Drawing for the job (mm, zero at the part's lowest x, y, z). Give positions to 0.01 mm unless a question says otherwise; leave off trailing zeros. Order: outer loops, then holes, each group sorted by start corner. A loop starts at its lowest first (then second) coordinate and runs counter-clockwise, first axis right, second up. Notation, with made-up numbers: (40, -2.5) - (70, -2.5) arc R23 cw to (70, 18.5) - close; hole circle Ø10 at (85.5, 12.25). An arc over 180 degrees is marked (long way). Use a Markdown table: item, result.
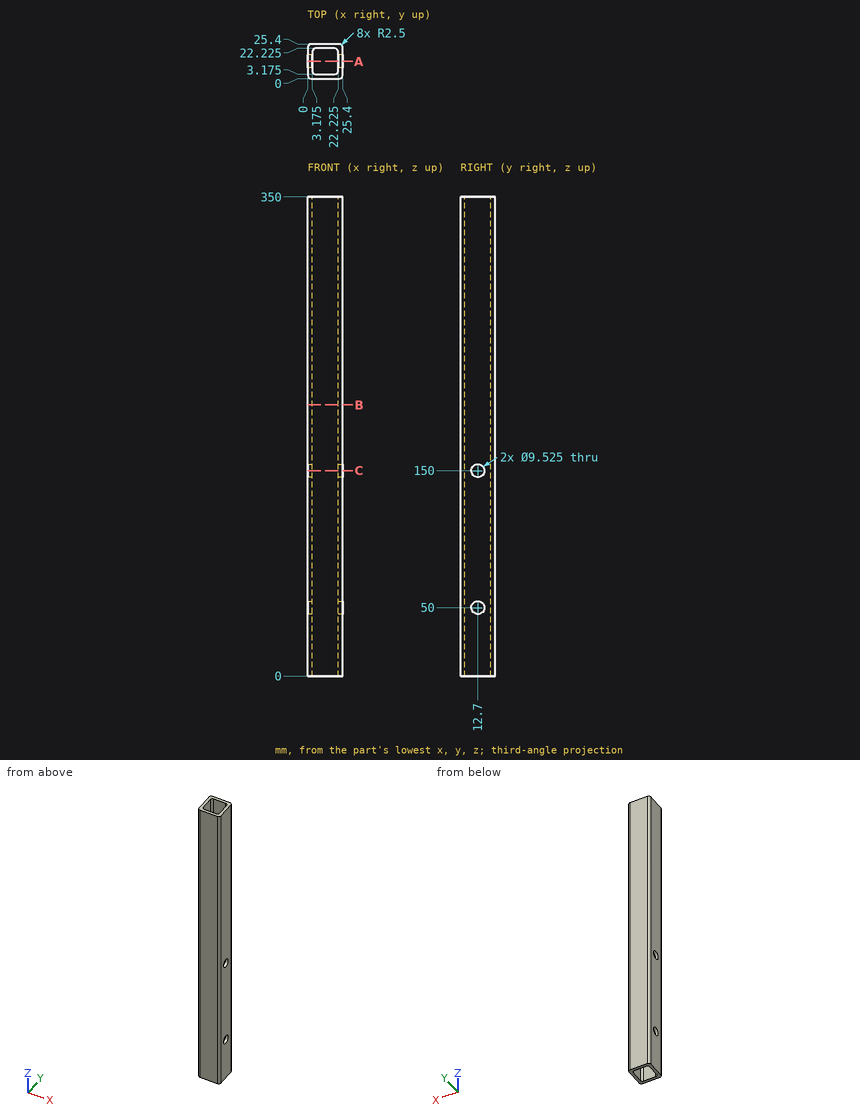
1) Slice it at B-B (z = 198). Write the cut outline in (x, y) (3 decimals), and give its area (3 significant figures).
Computed:
| item | result |
|---|---|
| outline | (0, 2.5) arc R2.5 ccw to (2.5, 0) - (22.9, 0) arc R2.5 ccw to (25.4, 2.5) - (25.4, 22.9) arc R2.5 ccw to (22.9, 25.4) - (2.5, 25.4) arc R2.5 ccw to (0, 22.9) - close; hole (3.175, 5.675) arc R2.5 ccw to (5.675, 3.175) - (19.725, 3.175) arc R2.5 ccw to (22.225, 5.675) - (22.225, 19.725) arc R2.5 ccw to (19.725, 22.225) - (5.675, 22.225) arc R2.5 ccw to (3.175, 19.725) - close |
| area | 282 mm² |
2) Slice it at C-C (z = 150). Write the cut outline in (x, y) (1 decimal), and give its area (3 significant figures).
Computed:
| item | result |
|---|---|
| outline | (0, 2.5) arc R2.5 ccw to (2.5, 0) - (22.9, 0) arc R2.5 ccw to (25.4, 2.5) - (25.4, 7.9) - (22.2, 7.9) - (22.2, 5.7) arc R2.5 cw to (19.7, 3.2) - (5.7, 3.2) arc R2.5 cw to (3.2, 5.7) - (3.2, 7.9) - (0, 7.9) - close; (0, 17.5) - (3.2, 17.5) - (3.2, 19.7) arc R2.5 cw to (5.7, 22.2) - (19.7, 22.2) arc R2.5 cw to (22.2, 19.7) - (22.2, 17.5) - (25.4, 17.5) - (25.4, 22.9) arc R2.5 ccw to (22.9, 25.4) - (2.5, 25.4) arc R2.5 ccw to (0, 22.9) - close |
| area | 222 mm² |
3) Slice it at A-A (y = 12.7). Write the cut outline in (x, z) (1 decimal).
Computed:
| item | result |
|---|---|
| outline | (0, 0) - (3.2, 0) - (3.2, 45.2) - (0, 45.2) - close; (0, 54.8) - (3.2, 54.8) - (3.2, 145.2) - (0, 145.2) - close; (0, 154.8) - (3.2, 154.8) - (3.2, 350) - (0, 350) - close; (22.2, 0) - (25.4, 0) - (25.4, 45.2) - (22.2, 45.2) - close; (22.2, 54.8) - (25.4, 54.8) - (25.4, 145.2) - (22.2, 145.2) - close; (22.2, 154.8) - (25.4, 154.8) - (25.4, 350) - (22.2, 350) - close |
4) Pin check, flat tip, straight feed: P1, Ø5.5, axis at y = 12.7, z = 150, coming from the -X side. Stop position of the tip, or through.
Computed:
| item | result |
|---|---|
| P1 | passes through |
5) Wall check: line 1 (X direction, y = 12.75, z = 180) (3 decimals); line 2 (Y direction, x = 24.4, z = 50). Give the ranges that are in metal, low to high. Write a range as from..to.
Computed:
| item | result |
|---|---|
| line 1 | x = 0..3.175, 22.225..25.4 |
| line 2 | y = 0.5..7.94, 17.46..24.9 |
